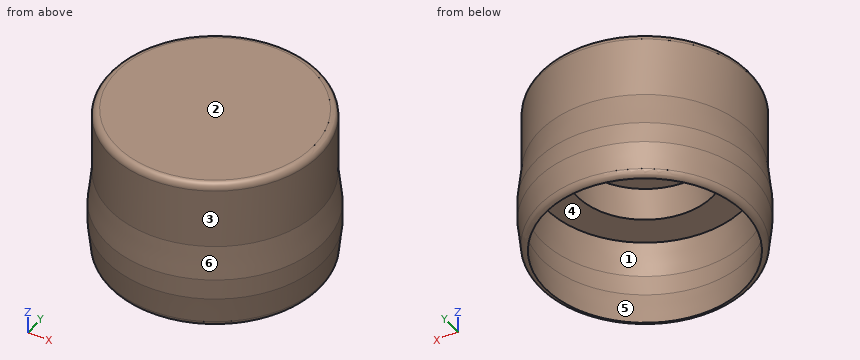
Autodesk Inventor part; units mm, degrees
ref_plane "YZ Plane" through (0, 0, 0) normal (1, 0, 0) x (0, 1, 0)
ref_plane "XZ Plane" through (0, 0, 0) normal (0, 1, 0) x (-1, 0, 0)
ref_plane "XY Plane" through (0, 0, 0) normal (0, 0, 1) x (1, 0, 0)
sketch "Sketch1" plane through (0, 0, 0) normal (1, 0, 0) x (0, 1, 0)
  line L0 (0, 0) -> (15.75, 0)
  line L1 (15.75, 0) -> (15.75, -10)
  line L2 (15.75, -10) -> (10.2, -10)
  line L3 (10.2, -10) -> (10.2, -5)
  line L4 (10.2, -5) -> (0, -5)
  line L5 (0, -5) -> (0, 0)
  point P0 (0, -2.5)
  point P1 (15.75, -5)
  point P2 (7.875, 0)
  dimension "d0" = 15.75
  dimension "d1" = 10.2
  dimension "d2" = 10
  dimension "d3" = 5
revolve "Revolution1" add sketch "Sketch1" angle 360 about axis through (0, 0, -5) along (0, 0, 1)
sketch "Sketch3" plane through (0, 0, 0) normal (1, 0, 0) x (0, 1, 0)
  line L0 (15.75, 0) -> (-15.75, 0)
  line L1 (15.75, -10) -> (-15.75, -10)
  line L2 (15.75, -10) -> (15.75, 0)
  line L3 (15.75, -10) -> (16.3, -15)
  line L4 (15.5, -15.0439) -> (14.9452, -10)
  line L5 (14.9452, -10) -> (15.75, -10)
  line L6 (0, -24.0479) -> (0, 4.008)
  line L7 (16.3, -15) -> (16.3, -18.0877)
  line L8 (15.5, -18.0439) -> (15.5, -15.0439)
  line L9 (15.5, -18.0439) -> (14.9548, -23.0003)
  line L10 (14.9548, -23.0003) -> (15.75, -23.0877)
  line L11 (15.75, -23.0877) -> (16.3, -18.0877)
  point P0 (0, 0)
  point P1 (0, 0)
  point P2 (15.2274, -20.5221)
  dimension "d14" = 0.8
  dimension "d15" = 16.3
  dimension "d16" = 5
  dimension "d19" = 0.8
  dimension "d21" = 3
  dimension "d22" = 5
  dimension "d25" = 0.8
revolve "Revolution2" add sketch "Sketch3" angle 360 about axis through (0, 0, -10) along (0, 0, 1) contours L3 L7 L11 L10 L9 L8 L4 L1
fillet "Fillet2" radius 1 2 edges at (0, -15.75, 0) (0, -15.75, -23.0877)
properties part number "Spring_Top_3DPrint"
Design review of the part built by this model. Coordinates are the model's own, in mm. Face numbers are marked on the shaded views. A direction names the side the tool comes from. Coordinates: 2 decimals unless noted, no trailing zeros. Loops run counter-clockwise (first coordinate to the right, second up) from the corner with the lowest first, then second, coordinate; pieces in that order, holes last.
Item 1: Add section A-A (y = 0). Write out the cut boundary in (x, z).
Completed:
outline: (-16.3, -18.09) - (-15.86, -22.11) arc R1 ccw to (-14.95, -23) - (-15.5, -18.04) - (-15.5, -15.04) - (-14.95, -10) - (-10.2, -10) - (-10.2, -5) - (10.2, -5) - (10.2, -10) - (14.95, -10) - (15.5, -15.04) - (15.5, -18.04) - (14.95, -23) arc R1 ccw to (15.86, -22.11) - (16.3, -18.09) - (16.3, -15) - (15.75, -10) - (15.75, -1) arc R1 ccw to (14.75, 0) - (-14.75, 0) arc R1 ccw to (-15.75, -1) - (-15.75, -10) - (-16.3, -15) - close
Item 2: Add section B-B (z = -15.5). Write out the cut boundary in (x, y), and give its area (3 significant figures).
Completed:
outline: circle Ø32.6 at (0, 0); hole circle Ø31 at (0, 0)
area: 79.9 mm2
Item 3: For the marked faces 4, 5 and 6, list the 3-axis set-ups (+Z, -Z, +X, -X, +Y, -Y) from which the entire face can be reached by the end or side of a thin tool; tool diameter is ignored.
Completed:
face 4: -Z
face 5: none
face 6: +Z
Item 4: Clearance check with flat-ended pins moving along their axes: pin 1 (1 mm diameter, centred on y = 7, z = -3.5, fed in from -X); pin 2 (4 mm diameter, centred on x = -13, z = -4, fed in from -Y); pin 3 (3 mm diameter, centred on x = -12, z = -6, fed in from +Y); pin 4 (4 mm diameter, centred on x = -9, y = 8.5, fed in from +Z). State where each tip first meets the part, or that it passes through.
Completed:
pin 1: stops at x = -14.35
pin 2: stops at y = -11.27
pin 3: stops at y = 11.74
pin 4: stops at z = 0
Item 5: Add section D-D (z = -8.25). Write out the cut boundary in (x, y), and give its area (3 significant figures).
Completed:
outline: circle Ø31.5 at (0, 0); hole circle Ø20.4 at (0, 0)
area: 452 mm2
Item 6: Wall thickness on L1, parallel to X at y = 0, z = -7.2; L2, parallel to Y at x = 0, z = -15.8: over which ranges is each line inside the solid? List them lowest first.
Completed:
L1: x = -15.75 to -10.2, 10.2 to 15.75
L2: y = -16.3 to -15.5, 15.5 to 16.3
Item 7: Draft analysis for pull direction X (two halves, no side actions). For the marked faces 1, 2 and 3, state which applies: pulls with the +X half, pulls with the -X half, needs draft (parallel to the pull), parting line crosses it, or undercut.
Completed:
face 1: undercut
face 2: needs draft
face 3: parting line crosses it
